from build123d import *

# Parameters (mm, degrees)
SKETCH1_W           = 32.03
SKETCH1_H           = 20.25
BOSS_EXTRUDE1_DEPTH = 42.5
SKETCH2_W           = 32.03
SKETCH2_H           = 20.25
SKETCH2_W_2         = 22.03
SKETCH2_H_2         = 18.42
BOSS_EXTRUDE2_DEPTH = 2
CUT_EXTRUDE1_DEPTH  = 25.25
FILLET1_R           = 3
SKETCH6_R           = 2.6
CUT_EXTRUDE3_DEPTH  = 25.25
CHAMFER2_SIZE       = 2
BOSS_EXTRUDE3_REACH = 24.25
CUT_EXTRUDE4_REACH  = 38.03
SKETCH8_W           = 38.5
SKETCH8_H           = 20.25
FILLET2_R           = 1


with BuildPart() as part:
    # Sketch1 → Boss-Extrude1 (new body)
    with BuildSketch(Plane.XY):
        Polygon((26.409748294, 13.899702025), (26.409748294, -6.350297975), (29.409748294, -6.350297975), (29.409748294, -8.350297975), (-9.620251706, -8.350297975), (-9.620251706, 15.899702025), (46.409748294, 15.899702025), (46.409748294, 13.899702025), align=None)
        with Locations((8.394748294, 3.774702025)):
            Rectangle(SKETCH1_W, SKETCH1_H, mode=Mode.SUBTRACT)
    extrude(amount=BOSS_EXTRUDE1_DEPTH)

    # Sketch2 → Boss-Extrude2 (add)
    with BuildSketch(Plane.XY.offset(42.5)):
        with Locations((8.394748294, 3.774702025)):
            Rectangle(SKETCH2_W, SKETCH2_H)
        with Locations((8.894748294, 3.422592454)):
            Rectangle(SKETCH2_W_2, SKETCH2_H_2, mode=Mode.SUBTRACT)
    extrude(amount=-BOSS_EXTRUDE2_DEPTH)

    # Sketch3 → Cut-Extrude1 (cut, through all)
    with BuildSketch(Plane.XZ.offset(8.350297975)):
        Polygon((-9.620251706, 0), (-9.620251706, 21.25), (11.629748294, 0), align=None)
    extrude(amount=-CUT_EXTRUDE1_DEPTH, mode=Mode.SUBTRACT)

    # Fillet1
    fillet1_edges = [part.edges().sort_by_distance(p)[0] for p in [
        (46.409748294, 14.899702025, 0),
        (29.409748294, -7.350297975, 0),
        (46.409748294, 14.899702025, 42.5),
        (29.409748294, -7.350297975, 42.5),
    ]]
    fillet(fillet1_edges, radius=FILLET1_R)

    # Sketch6 → Cut-Extrude3 (cut, through all)
    with BuildSketch(Plane(origin=(0, 15.899702025, 0), x_dir=(1, 0, 0), z_dir=(0, 1, 0))):
        with Locations((36.409748294, -33.25)):
            Circle(SKETCH6_R)
        with Locations((36.409748294, -9.25)):
            Circle(SKETCH6_R)
    extrude(amount=-CUT_EXTRUDE3_DEPTH, mode=Mode.SUBTRACT)

    # Chamfer2
    chamfer2_edges = [part.edges().sort_by_distance(p)[0] for p in [
        (1.004748294, 15.899702025, 10.625),
        (-9.620251706, 15.899702025, 31.875),
        (1.004748294, -8.350297975, 10.625),
        (-9.620251706, -8.350297975, 31.875),
    ]]
    chamfer(chamfer2_edges, length=CHAMFER2_SIZE)

    # Sketch7 → Boss-Extrude3 (add, up to next)
    with BuildSketch(Plane(origin=(0, -6.350297975, 0), x_dir=(1, 0, 0), z_dir=(0, 1, 0)), mode=Mode.PRIVATE) as boss_extrude3_sk1:
        Polygon((24.409748294, 0), (11.629748294, 0), (-7.620251706, -19.25), (-7.620251706, -22.078427125), (12.458175419, -2), (24.409748294, -2), align=None)
    boss_extrude3_tool1 = extrude(boss_extrude3_sk1.sketch, amount=BOSS_EXTRUDE3_REACH, mode=Mode.PRIVATE) - part.part
    add(boss_extrude3_tool1.solids().sort_by_distance((18.019748, -6.350298, 0.389022))[0])

    # Sketch8 → Cut-Extrude4 (cut, up to next)
    with BuildSketch(Plane(origin=(26.409748294, 0, 0), x_dir=(0, 0, -1), z_dir=(1, 0, 0)), mode=Mode.PRIVATE) as cut_extrude4_sk1:
        with Locations((-21.25, 3.774702025)):
            Rectangle(SKETCH8_W, SKETCH8_H)
    cut_extrude4_tool1 = extrude(cut_extrude4_sk1.sketch, amount=-CUT_EXTRUDE4_REACH, mode=Mode.PRIVATE) & part.part
    add(cut_extrude4_tool1.solids().sort_by_distance((26.409748, 3.774702, 21.25))[0], mode=Mode.SUBTRACT)

    # Fillet2
    fillet2_edges = [part.edges().sort_by_distance(p)[0] for p in [
        (26.409748294, 13.899702025, 1),
        (26.409748294, -6.350297975, 1),
        (26.409748294, 13.899702025, 41.5),
        (26.409748294, -6.350297975, 41.5),
    ]]
    fillet(fillet2_edges, radius=FILLET2_R)


solid = part.part
Part model, mm, in its own coordinate system. A direction names the side the tool comes from. Coordinates: 2 decimals unless noted, no trailing zeros. Order: outer loops, then holes, each group sorted by start corner. A loop starts at its lowest first (then second) coordinate and runs counter-clockwise, first axis right, second up. Notation, with made-up numbers: M 69.25,-3 L 74.25,-3 A12 cw 74.25,11 Z; hole C 51,87.25 d2. An arc over 180 degrees is marked long. Use a Markdown table: item, result.
(1) Cut at B-B on z = 33.25. Write the cut outline in (x, y).
A:
| item | result |
|---|---|
| outline | M -9.62,-6.35 L -7.62,-8.35 L 29.41,-8.35 L 29.41,-6.35 L -7.62,-6.35 L -7.62,13.9 L 33.81,13.9 L 33.81,15.9 L -7.62,15.9 L -9.62,13.9 Z; M 39.01,13.9 L 46.41,13.9 L 46.41,15.9 L 39.01,15.9 Z |
(2) Tool access for faces 1 (the flat face through (26.41, 4, 41)), 2 (the flat face through (11, -6.35, 26)), 3 (the cylindrical face through (28.55, -7.2, 0.9)), 4 (the flat face through (46.41, 15, 21)), 5 (the flat face through (19.91, 3, 42)): list every direction of +Z, -Z, +X, -X, +Y, -Y with a clear straight run to the whole face (end or side of a thin tool).
A:
| item | result |
|---|---|
| face 1 | +Z, -Z, +X |
| face 2 | +X |
| face 3 | -Z, +X, -Y |
| face 4 | +Z, -Z, +X, +Y, -Y |
| face 5 | +Z |
(3) Cut at D-D on z = 25.5. Write the cut outline in (x, y).
A:
| item | result |
|---|---|
| outline | M -9.62,-6.35 L -7.62,-8.35 L 29.41,-8.35 L 29.41,-6.35 L -7.62,-6.35 L -7.62,13.9 L 46.41,13.9 L 46.41,15.9 L -7.62,15.9 L -9.62,13.9 Z |
(4) Pull direction X, two halves, no side cores. Call faces 6 (the flat face through (-9.62, 4, 32)), 7 (the flat face through (-2.12, 3, 42)), 8 (the flat face through (11, -8.35, 26)): released by +X, released by -X, zero draft, split by the parting line, or undercut.
A:
| item | result |
|---|---|
| face 6 | released by -X |
| face 7 | undercut |
| face 8 | zero draft |
(5) Probe L1, parallel to Y at x = 28.5, z = 35; L2, parallel to Y at x = 35.5, z = 2; L3, parallel to Z at x = 20, y = 10.75. List the from-to ranges inside material, lowest first.
A:
| item | result |
|---|---|
| L1 | y = -8.35 to -6.35, 13.9 to 15.9 |
| L2 | y = 13.9 to 15.9 |
| L3 | z = 0 to 2, 40.5 to 42.5 |
(6) Cut at C-C on x = 22.5. Write the cut outline in (y, z), then the cut area to 3 significant figures.
A:
| item | result |
|---|---|
| outline | M -8.35,0 L 15.9,0 L 15.9,42.5 L -8.35,42.5 Z; hole M -6.35,2 L 13.9,2 L 13.9,40.5 L -6.35,40.5 Z |
| area | 251 mm^2 |
(7) Flat gauge pins, fed straight in: pin 1 (1 mm diameter, centred on y = -7, z = 21, fed in from +X); pin 2 (8 mm diameter, centred on y = 9.5, z = 38, fed in from +X); pin 3 (4 mm diameter, centred on y = 8, z = 26.5, fed in from +X); pin 4 (4 mm diameter, centred on x = 1, z = 7, fed in from -Y). Where does each tip first touch, or does it go through?
A:
| item | result |
|---|---|
| pin 1 | stops at x = 29.41 |
| pin 2 | stops at x = 26.41 |
| pin 3 | stops at x = -7.62 |
| pin 4 | passes through |
(8) Cut at A-A on y = 10.5. Write the cut outline in (x, z).
A:
| item | result |
|---|---|
| outline | M -9.62,21.25 L 11.63,0 L 26.41,0 L 26.41,2 L 12.46,2 L -7.62,22.08 L -7.62,40.5 L -2.12,40.5 L -2.12,42.5 L -9.62,42.5 Z; M 19.91,40.5 L 26.41,40.5 L 26.41,42.5 L 19.91,42.5 Z |
